```python
from build123d import *

# Parameters (mm, degrees)
BASE_DEPTH           = 28.575
BACK_PLATE_DEPTH     = 2.54
SKETCH4_R            = 2.413
MOUNTING_HOLES_DEPTH = 7.35


with BuildPart() as part:
    # Sketch2 → Base (new body)
    with BuildSketch(Plane.XY):
        with BuildLine():
            Line((13.335, -19.05), (0, -19.05))
            Line((0, -19.05), (0, -25.4))
            Line((0, -25.4), (36.83, -25.4))
            Line((36.83, -25.4), (36.83, -19.05))
            Line((36.83, -19.05), (27.94, -19.05))
            ThreePointArc((27.94, -19.05), (26.143948776, -18.306051224), (25.4, -16.51))
            Line((25.4, -16.51), (25.4, 0))
            Line((25.4, 0), (15.875, 0))
            Line((15.875, 0), (15.875, -6.35))
            Line((15.875, -6.35), (18.415, -6.35))
            ThreePointArc((18.415, -6.35), (20.32, -8.255), (18.415, -10.16))
            Line((18.415, -10.16), (15.875, -10.16))
            Line((15.875, -10.16), (15.875, -16.51))
            ThreePointArc((15.875, -16.51), (15.131051224, -18.306051224), (13.335, -19.05))
        make_face()
    base = extrude(amount=BASE_DEPTH)

    # Sketch5 → Back Plate (add)
    with BuildSketch(Plane.XY.offset(28.575)):
        with BuildLine():
            Line((0, -25.4), (36.83, -25.4))
            Line((36.83, -25.4), (36.83, -19.05))
            Line((36.83, -19.05), (27.94, -19.05))
            ThreePointArc((27.94, -19.05), (26.143948776, -18.306051224), (25.4, -16.51))
            Line((25.4, -16.51), (25.4, 0))
            Line((25.4, 0), (15.875, 0))
            Line((15.875, 0), (15.875, -6.35))
            Line((15.875, -6.35), (15.875, -10.16))
            Line((15.875, -10.16), (15.875, -16.51))
            ThreePointArc((15.875, -16.51), (15.131051224, -18.306051224), (13.335, -19.05))
            Line((13.335, -19.05), (0, -19.05))
            Line((0, -19.05), (0, -25.4))
        make_face()
    back_plate = extrude(amount=BACK_PLATE_DEPTH)

    # Sketch4 → Mounting Holes (cut, through all)
    with BuildSketch(Plane(origin=(0, -19.05, 0), x_dir=(1, 0, 0), z_dir=(0, 1, 0))):
        with Locations((32.385, -15.5575)):
            Circle(SKETCH4_R)
    mounting_holes = extrude(amount=-MOUNTING_HOLES_DEPTH, mode=Mode.SUBTRACT)

    # Mirror 2: Base, Back Plate, Mounting Holes across plane
    add(base.mirror(Plane(origin=(0, 0, 0), x_dir=(0, 0, 1), z_dir=(1, 0, 0))))
    add(back_plate.mirror(Plane(origin=(0, 0, 0), x_dir=(0, 0, 1), z_dir=(1, 0, 0))))
    add(mounting_holes.mirror(Plane(origin=(0, 0, 0), x_dir=(0, 0, 1), z_dir=(1, 0, 0))), mode=Mode.SUBTRACT)


solid = part.part
```
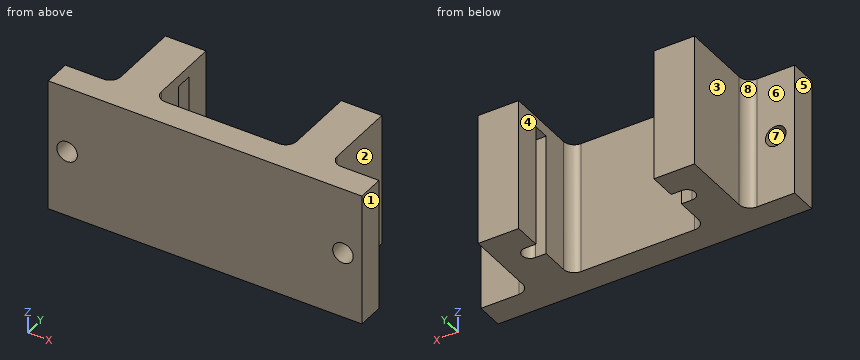
Input: part model. Units: mm. Frame: model coordinates. Face numbers are marked on the shaded views. A direction names the side the tool comes from. Coordinates: 2 decimals unless noted, no trailing zeros. Write each loop counter-clockwise with the first axis right and the second up, starting at its lowest first coordinate (ties: lowest second). Pieces come first, ordered by that corner, then holes.
1) Section D-D on z = 5. Output: boundary loops of the cut face in (x, y) (3 decimals).
2) Section B-B on x = -17.5. Output: boundary loops of the cut face in (y, z) (3 decimals), and give its area (3 significant figures).
3) Mould query, pull axis X, two halves, no side actions, for the marked faces 6, 7 and 8. Classes: pulls with the +X half, pulls with the -X half, needs draft (parallel to the pull), parting line crosses it, or undercut.
4) Section C-C on z = 17. State how many separate pieces and enclosed holes the cut face has, and give its area (3 significant figures).
5) Section A-A on y = -15.75. Output: boundary loops of the cut face in (x, z) (3 decimals).
6) Material intervals for line 1 along X through (y, z) = (-2.75, 24.5) (3 decimals); line 2 along Y through (x, z) = (0, 12); line 3 along Z through (x, y) = (-34, -23.75) (3 decimals), sorted ascending.
7) Set-up query: the marked faces 1, 2, 3, 4 and 5. Return all of +Z, -Z, +X, -X, +Y, -Y with unobstructed straight access to the full face (end or side cutting, diameter ignored); none if empty.
8) Pin query (flat end, axial travel): pin 1 Ø2 at (y, z) = (-15, 5.5) entering from -X; pin 2 Ø2.5 at (x, z) = (-31.5, 8.5) entering from +Y; pin 3 Ø5 at (y, z) = (-11.5, 11) entering from +X. Return the tip coordinate at first contact, or that it passes through.
Check result:
1. outline: (-36.83, -25.4) - (36.83, -25.4) - (36.83, -19.05) - (27.94, -19.05) arc R2.54 cw to (25.4, -16.51) - (25.4, 0) - (15.875, 0) - (15.875, -6.35) - (18.415, -6.35) arc R1.905 cw to (18.415, -10.16) - (15.875, -10.16) - (15.875, -16.51) arc R2.54 cw to (13.335, -19.05) - (-13.335, -19.05) arc R2.54 cw to (-15.875, -16.51) - (-15.875, -10.16) - (-18.415, -10.16) arc R1.905 cw to (-18.415, -6.35) - (-15.875, -6.35) - (-15.875, 0) - (-25.4, 0) - (-25.4, -16.51) arc R2.54 cw to (-27.94, -19.05) - (-36.83, -19.05) - close
2. outline: (-25.4, 0) - (-10.16, 0) - (-10.16, 28.575) - (-6.35, 28.575) - (-6.35, 0) - (0, 0) - (0, 31.115) - (-25.4, 31.115) - close
2. area: 681 mm2
3. face 6: needs draft
3. face 7: undercut
3. face 8: pulls with the -X half
4. separate pieces: 3
4. enclosed holes: 0
4. area: 756 mm2
5. outline: (-25.4, 0) - (-15.875, 0) - (-15.875, 31.115) - (-25.4, 31.115) - close; (15.875, 0) - (25.4, 0) - (25.4, 31.115) - (15.875, 31.115) - close
6. line 1: x = -25.4 to -15.875, 15.875 to 25.4
6. line 2: y = -25.4 to -19.05
6. line 3: z = 0 to 13.765, 17.35 to 31.115
7. face 1: +Z, -Z, +X, +Y, -Y
7. face 2: +Z, -Z, +X, +Y
7. face 3: +Z, -Z, -X, +Y
7. face 4: +Z, -Z, +Y
7. face 5: +Z, -Z, -X, +Y, -Y
8. pin 1: stops at x = -25.4
8. pin 2: stops at y = -19.05
8. pin 3: stops at x = 25.4
